Autodesk Inventor part; units mm, degrees
ref_plane "Work Plane1" through (0, 3, 0) normal (0, 1, 0) x (-1, 0, 0)
ref_plane "YZ Plane" through (0, 0, 0) normal (1, 0, 0) x (0, 1, 0)
ref_plane "XY Plane" through (0, 0, 0) normal (0, 0, 1) x (1, 0, 0)
sketch "Sketch1" plane through (0, 0, 0) normal (0, 0, 1) x (1, 0, 0)
  circle A0 centre (0, 0) radius 22.5
  dimension "d0" = 45
extrude "Extrusion1" add sketch "Sketch1" along normal mid plane 5
sketch "Sketch2" plane through (0, 0, 2.5) normal (0, 0, 1) x (1, 0, 0)
  circle A0 centre (0, 0) radius 4
  circle A1 centre (0, 15) radius 4
  circle A2 centre (-13.5, -7.5) radius 4.5
  circle A3 centre (13.5, -7.5) radius 4.5
  dimension "d3" = 8
  dimension "d4" = 15
  dimension "d5" = 8
  dimension "d6" = 7.5
  dimension "d7" = 13.5
  dimension "d8" = 13.5
  dimension "d9" = 9
  dimension "d10" = 9
extrude "Extrusion2" cut sketch "Sketch2" against normal up to surface (5 mm away)
fillet "Fillet1" radius 0.5 2 edges at (-22.5, 0, 2.5) (-22.5, 0, -2.5)
ref_plane "Work Plane1" through (0, 3, 0) normal (0, 1, 0) x (-1, 0, 0)
sketch "Sketch3" plane through (0, 3, 0) normal (0, 1, 0) x (-1, 0, 0)
  line L0 (-4, 2.5) -> (4, 2.5)
  line L1 (4, -2.5) -> (-4, -2.5)
  line L2 (22.5, 2) -> (-22.5, 2)
  line L3 (-22.5, -2) -> (22.5, -2)
  line L4 (-22.5, -2) -> (-22.5, 2)
  line L5 (22.5, -2) -> (22.5, 2)
  point P0 (0, 0)
  point P1 (0, 0)
  point P2 (-22.5, 0)
  point P3 (0, -2)
hole "Hole1" at (0, 3, 0) direction (0, 1, 0) diameter 3 end through all
equation "\"d10\" = d9"
equation "\"d11\" = d10"
properties part number "201 part 3" material "Aluminum 6061-AHC"
Can you work these out from the model? Positions are in its coordinate system, mm. A direction names the side the tool comes from. Give positions to 0.01 mm unless a question says otherwise; leave off trailing zeros. Write each loop counter-clockwise with the first axis right and the second up, starting at its lowest first coordinate (ties: lowest second). Pieces come first, ordered by that corner, then holes. Notation, with made-up numbers: (72.5, 73) -> (109.5, 73) arc R14 ccw to (109.5, 91) -> close; hole circle Ø6 at (78, -8). An arc over 180 degrees is marked (long way). One line per item, written item: value.
Q1. Imagine slicing it at A-A on y = 0. Please give me the cut outline in (x, z).
Results found:
outline: (-22.5, -2) arc R0.5 ccw to (-22, -2.5) -> (-4, -2.5) -> (-4, 2.5) -> (-22, 2.5) arc R0.5 ccw to (-22.5, 2) -> close; (4, -2.5) -> (22, -2.5) arc R0.5 ccw to (22.5, -2) -> (22.5, 2) arc R0.5 ccw to (22, 2.5) -> (4, 2.5) -> close
Q2. Imagine slicing it at D-D on y = -7.5. Give the number of separate pieces and of enclosed holes in the cut face, and give its area (3 significant figures).
Results found:
separate pieces: 3
enclosed holes: 0
area: 122 mm^2
Q3. We'd pull the mould along Y, two halves only. Please class faces 3 (the face through (17.66, -9.22, 0.04)), 4 (the face through (10.382, 19.961, -0.028)), 5 (the face through (-0.07, 20.63, 1.5)): +Y half, -Y half, draft (parallel to the pull), parting line (faces both ways), or undercut.
Results found:
face 3: undercut
face 4: parting line
face 5: draft
Q4. Imagine slicing it at B-B on x = 0. Please give me the cut outline in (y, z).
Results found:
outline: (-22.5, -2) arc R0.5 ccw to (-22, -2.5) -> (-4, -2.5) -> (-4, 2.5) -> (-22, 2.5) arc R0.5 ccw to (-22.5, 2) -> close; (4, -2.5) -> (11, -2.5) -> (11, -1.5) -> (4, -1.5) -> close; (4, 1.5) -> (11, 1.5) -> (11, 2.5) -> (4, 2.5) -> close; (19, -2.5) -> (22, -2.5) arc R0.5 ccw to (22.5, -2) -> (22.5, -1.5) -> (19, -1.5) -> close; (19, 1.5) -> (22.5, 1.5) -> (22.5, 2) arc R0.5 ccw to (22, 2.5) -> (19, 2.5) -> close
Q5. Imagine slicing it at C-C on z = 0. Please give me the cut outline in (x, y), and give its area (3 significant figures).
Results found:
outline: (-1.5, 3.71) -> (-1.5, 11.29) arc R4 cw to (-1.5, 18.71) -> (-1.5, 22.45) arc R22.5 ccw (long way) to (1.5, 22.45) -> (1.5, 18.71) arc R4 cw to (1.5, 11.29) -> (1.5, 3.71) arc R4 cw (long way) to start; hole circle Ø9 at (-13.5, -7.5); hole circle Ø9 at (13.5, -7.5)
area: 1,330 mm^2
Q6. Which directions (+Z, -Z, +X, -X, +Y, -Y) give clear straight access to the entire face, cutting with the end or side of a thin tool? Please do faces 1 (the face through (-0.07, 7.55, 1.5)), 2 (the face through (5, 0, 2.5)).
Results found:
face 1: +Y
face 2: +Z, +X, -X, +Y, -Y
Q7. Please list where these lines run through material, in increasing order: line 1 (Y direction, x = -13.5, z = -0.9); line 2 (X direction, y = -5, z = -0.55); line 3 (Z direction, x = 0, y = 5.75). Write a range as [from, to].
Results found:
line 1: y = [-18, -12], [-3, 18]
line 2: x = [-21.94, -17.24], [-9.76, 9.76], [17.24, 21.94]
line 3: z = [-2.5, -1.5], [1.5, 2.5]
Q8. For P1, Ø1, axis at y = -1.5, z = 0.5, coming from the +X side; P2, Ø1, axis at y = 13.5, z = 1.5, coming from the -X side; P3, Ø2.5, axis at x = 0, z = 0, coming from the -Y side; P4, Ø5, axis at x = 0, y = 15, coming from the -Z side, each with a flat end and sliding along its axis, tell me the tip position at first contact or that it passes through.
Results found:
P1: stops at x = 22.48
P2: stops at x = -18.36
P3: stops at y = -22.5
P4: passes through
